```python
from build123d import *

# Parameters (mm, degrees)
SKETCH1_R           = 3.325
BOSS_EXTRUDE2_DEPTH = 38.1
BOSS_EXTRUDE3_REACH = 84.488
SKETCH6_W           = 38.1
SKETCH6_H           = 25.4
SKETCH10_R          = 2
CUT_EXTRUDE6_DEPTH  = 8
CHAMFER1_SIZE       = 1
CUT_EXTRUDE9_DEPTH  = 6.3
FILLET3_R           = 1
SKETCH16_R          = 2
CUT_EXTRUDE10_DEPTH = 5


with BuildPart() as part:
    # Sketch1 → Boss-Extrude2 (new body)
    with BuildSketch(Plane(origin=(0, 0, 0), x_dir=(0, 0, -1), z_dir=(1, 0, 0))):
        with BuildLine():
            Line((0, 22.75), (0, 0))
            ThreePointArc((0, 0), (12.7, -12.7), (25.4, 0))
            ThreePointArc((25.4, 0), (38.1, -12.7), (50.8, 0))
            Line((50.8, 0), (64, 8.107573416))
            Line((64, 8.107573416), (64, 22.75))
            Line((64, 22.75), (0, 22.75))
        make_face()
        with Locations(Location((38.1, 0, 0), (0, 0, 180))):
            Circle(SKETCH1_R, mode=Mode.SUBTRACT)
        with Locations(Location((12.7, 0, 0), (0, 0, 180))):
            Circle(SKETCH1_R, mode=Mode.SUBTRACT)
    extrude(amount=BOSS_EXTRUDE2_DEPTH)

    # Sketch6 → Boss-Extrude3 (add, up to next)
    with BuildSketch(Plane(origin=(0, -12.7, 0), x_dir=(-1, 0, 0), z_dir=(0, -1, 0)), mode=Mode.PRIVATE) as boss_extrude3_sk1:
        with Locations((-19.05, 25.4)):
            Rectangle(SKETCH6_W, SKETCH6_H)
    boss_extrude3_tool1 = extrude(boss_extrude3_sk1.sketch, amount=-BOSS_EXTRUDE3_REACH, mode=Mode.PRIVATE) - part.part
    add(boss_extrude3_tool1.solids().sort_by_distance((19.05, -12.7, -25.4))[0])

    # Sketch10 → Cut-Extrude6 (cut)
    with BuildSketch(Plane.XY):
        with Locations((9.525, 14.153125)):
            Circle(SKETCH10_R)
        with Locations((28.575, 14.153125)):
            Circle(SKETCH10_R)
    extrude(amount=-CUT_EXTRUDE6_DEPTH, mode=Mode.SUBTRACT)

    # Chamfer1
    chamfer1_edges = [part.edges().sort_by_distance(p)[0] for p in [
        (0, 0, -16.025),
        (0, 0, -41.425),
        (38.1, 0, -41.425),
        (38.1, 0, -16.025),
    ]]
    chamfer(chamfer1_edges, length=CHAMFER1_SIZE)

    # Sketch15 → Cut-Extrude9 (cut)
    with BuildSketch(Plane(origin=(0, 22.75, 0), x_dir=(1, 0, 0), z_dir=(0, 1, 0))):
        Polygon((12.5, 50.995), (0, 50.995), (0, 48.925), (15.26, 48.925), (15.26, 64), (12.5, 64), align=None)
        Polygon((25.6, 64), (22.84, 64), (22.84, 48.925), (38.1, 48.925), (38.1, 50.995), (25.6, 50.995), align=None)
    extrude(amount=-CUT_EXTRUDE9_DEPTH, mode=Mode.SUBTRACT)

    # Fillet3
    fillet3_edges = [part.edges().sort_by_distance(p)[0] for p in [
        (15.26, 19.6, -48.925),
        (0, 16.45, -49.96),
        (0, 19.6, -48.925),
        (0, 19.6, -50.995),
        (12.5, 19.6, -50.995),
        (13.88, 16.45, -64),
        (12.5, 19.6, -64),
        (15.26, 19.6, -64),
        (38.1, 16.45, -49.96),
        (38.1, 19.6, -50.995),
        (38.1, 19.6, -48.925),
        (22.84, 19.6, -48.925),
        (24.22, 16.45, -64),
        (22.84, 19.6, -64),
        (25.6, 19.6, -64),
        (25.6, 19.6, -50.995),
    ]]
    fillet(fillet3_edges, radius=FILLET3_R)

    # Sketch16 → Cut-Extrude10 (cut)
    with BuildSketch(Plane(origin=(0, 22.75, 0), x_dir=(1, 0, 0), z_dir=(0, 1, 0))):
        with Locations(Location((32.1, 58, 0), (0, 0, 270))):
            Circle(SKETCH16_R)
        with BuildLine():
            ThreePointArc((21.05, 43.76), (20.464213562, 45.174213562), (19.05, 45.76))
            Line((19.05, 45.76), (19.05, 41.76))
            ThreePointArc((19.05, 41.76), (20.464213562, 42.345786438), (21.05, 43.76))
        make_face()
        with BuildLine():
            Line((19.05, 41.76), (19.05, 45.76))
            ThreePointArc((19.05, 45.76), (17.05, 43.76), (19.05, 41.76))
        make_face()
        with Locations(Location((6, 58, 0), (0, 0, 270))):
            Circle(SKETCH16_R)
    extrude(amount=-CUT_EXTRUDE10_DEPTH, mode=Mode.SUBTRACT)


solid = part.part
```
Input: part model. Units: mm. Frame: model coordinates. A direction names the side the tool comes from. Coordinates: 2 decimals unless noted, no trailing zeros. Write each loop counter-clockwise with the first axis right and the second up, starting at its lowest first coordinate (ties: lowest second). Pieces come first, ordered by that corner, then holes. Notation, with made-up numbers: M -39,32.25 L -3,32.25 A18 cw -3,65.25 Z; hole C 86.25,32.25 d10. An arc over 180 degrees is marked long. Use one line per item in the form item = value.
Q1. First-contact query: pin 1 (2 mm diameter, centred on x = 33.5, z = -46, fed in from -Y); pin 2 (1.2 mm diameter, centred on x = 31, z = -58.5, fed in from +Y); pin 3 (3 mm diameter, centred on x = 32.1, z = -58, fed in from -Y). Flat tips, straight axial feed; report the tip coordinate or a pass-through.
Answer below:
pin_1 = -10.66
pin_2 = 17.75
pin_3 = 3.5
Q2. Draft query along X for faces 5 (the face through (0, 9, -32)), 6 (the face through (19, 22.75, -25)), 7 (the face through (32, 17.75, -58)). Return one class per face: released by +X, released by -X, zero draft, split by the parting line, or undercut.
Answer below:
face_5 = released by -X
face_6 = zero draft
face_7 = undercut
Q3. Section B-B (y = -1). Count the separate pieces of the cut face and the enclosed holes in it, plus the area to 3 significant figures.
Answer below:
separate_pieces = 3
enclosed_holes = 0
area = 1,450 mm²
Q4. Section C-C (z = -58). Return loops of the section in (x, y).
Answer below:
outline = M 0,4.42 L 38.1,4.42 L 38.1,22.75 L 34.1,22.75 L 34.1,17.75 L 30.1,17.75 L 30.1,22.75 L 25.6,22.75 L 25.6,16.45 L 22.84,16.45 L 22.84,22.75 L 15.26,22.75 L 15.26,16.45 L 12.5,16.45 L 12.5,22.75 L 8,22.75 L 8,17.75 L 4,17.75 L 4,22.75 L 0,22.75 Z
Q5. Section D-D (y = -6). Return loops of the section in (x, z), plus the area to 3 significant figures.
Answer below:
outline = M 0,-49.29 L 38.1,-49.29 L 38.1,-1.51 L 0,-1.51 Z
area = 1,820 mm²
Q6. Section A-A (x = 6). Return loops of the section in (y, z) (3 decimals), plus the area to 3 significant figures.
Answer below:
outline = M -12.7,-38.1 A12.7 ccw 0,-50.8 L 8.108,-64 L 22.75,-64 L 22.75,-60 L 17.75,-60 L 17.75,-56 L 22.75,-56 L 22.75,-50.995 L 16.45,-50.995 L 16.45,-48.925 L 22.75,-48.925 L 22.75,0 L 0,0 A12.7 ccw -12.7,-12.7 Z; hole C 0,-38.1 d6.65; hole C 0,-12.7 d6.65
area = 1,880 mm²
Q7. Material intervals for probe 1 along X at (y, z) = (19, -58); probe 2 along Y at (x, z) = (23, -13); probe 3 along Z at (x, y) = (33, 1.5), sorted ascending. Write a range as from..to.
Answer below:
probe_1 = 0..4, 8..12.5, 15.26..22.84, 25.6..30.1, 34.1..38.1
probe_2 = -12.7..-3.31, 3.31..22.75
probe_3 = -53.24..-41.07, -35.13..-15.67, -9.73..0
Q8. Set-up query: faces 1 (the face through (32, 20, -50.995)), 2 (the face through (25.6, 20, -57)), 3 (the face through (6.601, 20.285, -56.092)), 4 (the face through (29, 14, -8)). Return all of +Z, -Z, +X, -X, +Y, -Y with unobstructed straight access to the full face (end or side cutting, diameter ignored); none if empty.
Answer below:
face_1 = +X, +Y
face_2 = -Z, +Y
face_3 = +Y
face_4 = +Z
